Work out the finished part from the listing and answer in its coordinate system (mm). Face numbers are marked on the shaded views. A direction names the side the tool comes from. Give positions to 0.01 mm unless a question says otherwise; leave off trailing zeros. Loops run counter-clockwise (first coordinate to the right, second up) from the corner with the lowest first, then second, coordinate; pieces in that order, holes last. Notation, with made-up numbers: (34.5, 75.5) - (41.5, 75.5) arc R25 cw to (41.5, 114.5) - close; hole circle Ø9 at (83, 79). An arc over 180 degrees is marked (long way). One line per question, with ' | ' between items. Start each with the question number.
1. Section B-B (x = 0) is taken. Determine the outline of the cut face in (y, z).
2. Section C-C (z = 2.15) is taken. Determine the outline of the cut face in (x, y), plus the area to 3 significant figures.
3. Section D-D (y = 4) is taken. Determine the outline of the cut face in (x, z).
4. For a pull along X with two mould halves and no side action, classify the marked faces 4, 5, 6 and 7 as released by +X, released by -X, zero draft, split by the parting line, or undercut.
5. Section A-A (y = -14.5) is taken. Determine the outline of the cut face in (x, z).
6. Find the intervals of material crossed by line 1 (X direction, y = -13, z = 0.9); line 2 (Y direction, x = 0, z = 2.95); line 3 (X direction, y = 1, z = 2.9), in increasing order.
7. Which of the six approach directions +Z, -Z, +X, -X, +Y, -Y give full straight-line access (tool end or side, diameter ignored) to the marked faces 1, 2 and 3?
8. Each of these flat-tipped pins is pushed along its axis until it touches: pin 1 (0.7 mm diameter, centred on x = 2.5, z = 3, fed in from +Y); pin 2 (1.1 mm diameter, centred on x = -0.5, z = 2.5, fed in from -Y); pin 3 (1.9 mm diameter, centred on x = -3.5, z = 2.5, fed in from +Y). Where does it stop, or does it pass through?
from build123d import *

# Parameters (mm, degrees)
SKETCH1_R           = 2.95
BOSS_EXTRUDE1_DEPTH = 5.9
CUT_EXTRUDE2_DEPTH  = 26.827504719


with BuildPart() as part:
    # Sketch1 → Boss-Extrude1 (new body)
    with BuildSketch(Plane.XY):
        with BuildLine():
            Line((-7.5, 0), (-7.5, -24))
            Line((-7.5, -24), (7.5, -24))
            Line((7.5, -24), (7.5, 0))
            ThreePointArc((7.5, 0), (0, 7.5), (-7.5, 0))
        make_face()
        Circle(SKETCH1_R, mode=Mode.SUBTRACT)
    extrude(amount=BOSS_EXTRUDE1_DEPTH)

    # Sketch3 → Cut-Extrude2 (cut, through all)
    with BuildSketch(Plane.XY.offset(5.9)):
        Polygon((-1.9, -24), (1.9, -24), (1.9, -19), (4.25, -19), (4.25, -16.1), (1.9, -16.1), (1.9, -12), (-1.9, -12), (-1.9, -16.1), (-4.25, -16.1), (-4.25, -19), (-1.9, -19), align=None)
    extrude(amount=-CUT_EXTRUDE2_DEPTH, mode=Mode.SUBTRACT)


solid = part.part
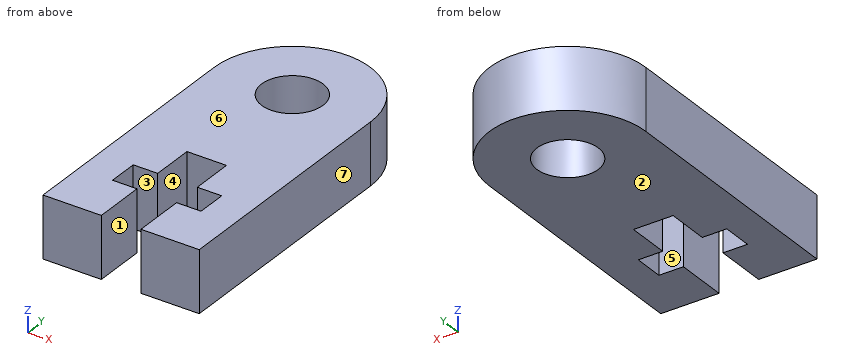
Conclusion:
1) outline: (-12, 0) - (-2.95, 0) - (-2.95, 5.9) - (-12, 5.9) - close; (2.95, 0) - (7.5, 0) - (7.5, 5.9) - (2.95, 5.9) - close
2) outline: (-7.5, -24) - (-1.9, -24) - (-1.9, -19) - (-4.25, -19) - (-4.25, -16.1) - (-1.9, -16.1) - (-1.9, -12) - (1.9, -12) - (1.9, -16.1) - (4.25, -16.1) - (4.25, -19) - (1.9, -19) - (1.9, -24) - (7.5, -24) - (7.5, 0) arc R7.5 ccw to (-7.5, 0) - close; hole circle Ø5.9 at (0, 0) | area: 362 mm²
3) outline: (-6.34, 0) - (6.34, 0) - (6.34, 5.9) - (-6.34, 5.9) - close
4) face 4: undercut | face 5: undercut | face 6: zero draft | face 7: released by +X
5) outline: (-7.5, 0) - (-1.9, 0) - (-1.9, 5.9) - (-7.5, 5.9) - close; (1.9, 0) - (7.5, 0) - (7.5, 5.9) - (1.9, 5.9) - close
6) line 1: -7.5 to -1.9, 1.9 to 7.5 | line 2: -12 to -2.95, 2.95 to 7.5 | line 3: -7.43 to -2.78, 2.78 to 7.43
7) face 1: +Z, -Z, -Y | face 2: -Z, +X, -X, +Y, -Y | face 3: +Z, -Z
8) pin 1: y = 7.19 | pin 2: y = -12 | pin 3: y = 7.05
